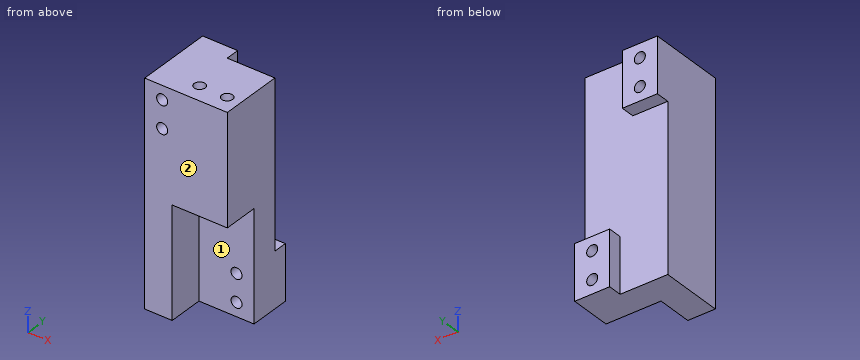
from build123d import *

# Parameters (mm, degrees)
SKETCH1_W           = 30
SKETCH1_H           = 80
BOSS_EXTRUDE1_DEPTH = 30
SKETCH2_W           = 12.7
SKETCH2_H           = 20
SKETCH2_R           = 2
BOSS_EXTRUDE2_DEPTH = 5
SKETCH3_R           = 2
CUT_EXTRUDE1_DEPTH  = 93.330926563
SKETCH4_W           = 20
SKETCH4_H           = 20
CUT_EXTRUDE2_DEPTH  = 40
SKETCH5_R           = 2
SKETCH5_W           = 30
SKETCH5_H           = 7.2
CUT_EXTRUDE3_DEPTH  = 93.330926563


with BuildPart() as part:
    # Sketch1 → Boss-Extrude1 (new body)
    with BuildSketch(Plane(origin=(0, 0, 0), x_dir=(1, 0, 0), z_dir=(0, 1, 0))):
        with Locations((-15, 40)):
            Rectangle(SKETCH1_W, SKETCH1_H)
    extrude(amount=BOSS_EXTRUDE1_DEPTH)

    # Sketch2 → Boss-Extrude2 (add)
    # profile 1 of 2: a face of its own
    with BuildSketch(Plane(origin=(0, 30, 0), x_dir=(1, 0, 0), z_dir=(0, 1, 0))):
        with Locations((-23.65, 10)):
            Rectangle(SKETCH2_W, SKETCH2_H)
        with Locations(Location((-23.65, 5, 0), (0, 0, 270))):
            Circle(SKETCH2_R, mode=Mode.SUBTRACT)
        with Locations(Location((-23.65, 15, 0), (0, 0, 270))):
            Circle(SKETCH2_R, mode=Mode.SUBTRACT)
    # profile 2 of 2: a face of its own
    with BuildSketch(Plane(origin=(0, 30, 0), x_dir=(1, 0, 0), z_dir=(0, 1, 0))):
        with Locations((-6.35, 70)):
            Rectangle(SKETCH2_W, SKETCH2_H)
        with Locations(Location((-6.35, 65, 0), (0, 0, 270))):
            Circle(SKETCH2_R, mode=Mode.SUBTRACT)
        with Locations(Location((-6.35, 75, 0), (0, 0, 270))):
            Circle(SKETCH2_R, mode=Mode.SUBTRACT)
    extrude(amount=BOSS_EXTRUDE2_DEPTH)

    # Sketch3 → Cut-Extrude1 (cut, through all)
    with BuildSketch(Plane(origin=(0, 35, 0), x_dir=(1, 0, 0), z_dir=(0, 1, 0))):
        with Locations(Location((-23.65, 15, 0), (0, 0, 270))):
            Circle(SKETCH3_R)
        with Locations(Location((-23.65, 5, 0), (0, 0, 270))):
            Circle(SKETCH3_R)
        with Locations(Location((-6.35, 75, 0), (0, 0, 270))):
            Circle(SKETCH3_R)
        with Locations(Location((-6.35, 65, 0), (0, 0, 270))):
            Circle(SKETCH3_R)
    extrude(amount=-CUT_EXTRUDE1_DEPTH, mode=Mode.SUBTRACT)

    # Sketch4 → Cut-Extrude2 (cut)
    with BuildSketch(Plane(origin=(0, 0, -80), x_dir=(-1, 0, 0), z_dir=(0, 0, -1))):
        with Locations((10, 10)):
            Rectangle(SKETCH4_W, SKETCH4_H)
    extrude(amount=-CUT_EXTRUDE2_DEPTH, mode=Mode.SUBTRACT)

    # Sketch5 → Cut-Extrude3 (cut, through all)
    with BuildSketch(Plane(origin=(0, 0, -80), x_dir=(-1, 0, 0), z_dir=(0, 0, -1))):
        with Locations((4.9, 13.6)):
            Circle(SKETCH5_R)
        with Locations((14.9, 13.6)):
            Circle(SKETCH5_R)
        with Locations((15, 3.6)):
            Rectangle(SKETCH5_W, SKETCH5_H)
    extrude(amount=-CUT_EXTRUDE3_DEPTH, mode=Mode.SUBTRACT)


solid = part.part
The model under review builds one solid part; all positions refer to its coordinate system, in mm. Face numbers are marked on the shaded views. A direction names the side the tool comes from. Give positions to 0.01 mm unless a question says otherwise; leave off trailing zeros. Write each loop counter-clockwise with the first axis right and the second up, starting at its lowest first coordinate (ties: lowest second). Pieces come first, ordered by that corner, then holes.
1. Add section C-C, the plane y = 13.6. Write out the cut boundary in (x, z), plus the area to 3 significant figures.
2. Add section D-D, the plane x = -14.9. Write out the cut boundary in (y, z).
3. For P1, Ø4, axis at x = -12.5, z = -48.5, coming from the +Y side; P2, Ø5, axis at y = 17, z = -31, coming from the +X side; P3, Ø5.5, axis at x = -8.5, y = 33, coming from the +Z side; P4, Ø2.5, axis at y = 33.5, z = -75, coming from the -X side, all flat-tipped, find the tip position at first contact; note any pin that passes through.
4. Wall thickness on L1, parallel to X at y = 19, z = -5; L2, parallel to Z at x = -7.5, y = 27.25; L3, parallel to X at y = 8.75, z = -62: over which ranges is each line inside the solid? List them lowest first.
5. Add section B-B, the plane z = -75. Write out the cut boundary in (x, y), plus the area to 4 significant figures.
6. Tool access review of the marked faces 1 and 2: name each direction out of +Z, -Z, +X, -X, +Y, -Y from which nothing blocks a thin tool from reaching the whole face with its end or side.
7. Add section A-A, the plane y = 25. Write out the cut boundary in (x, z), plus the area to 3 significant figures.
Worked answers:
1. outline: (-30, -80) - (-20, -80) - (-20, -40) - (-16.9, -40) - (-16.9, 0) - (-30, 0) - close; (-12.9, -40) - (-6.9, -40) - (-6.9, 0) - (-12.9, 0) - close; (-2.9, -40) - (0, -40) - (0, 0) - (-2.9, 0) - close; hole circle Ø4 at (-23.65, -15); hole circle Ø4 at (-23.65, -5)
1. area: 1,250 mm2
2. outline: (7.2, -40) - (11.6, -40) - (11.6, 0) - (7.2, 0) - close; (15.6, -40) - (20, -40) - (20, -80) - (30, -80) - (30, 0) - (15.6, 0) - close
3. P1: stops at y = 30
3. P2: stops at x = 0
3. P3: stops at z = -60
3. P4: stops at x = -12.7
4. L1: x = -30 to -25.65, -21.65 to 0
4. L2: z = -80 to -76.64, -73.36 to -66.64, -63.36 to 0
4. L3: x = -30 to -20
5. outline: (-30, 7.2) - (-20, 7.2) - (-20, 20) - (-8.35, 20) - (-8.35, 35) - (-12.7, 35) - (-12.7, 30) - (-30, 30) - close; (-4.35, 20) - (0, 20) - (0, 35) - (-4.35, 35) - close
5. area: 431.5 mm2
6. face 1: -Z, +X, -Y
6. face 2: +Z, -Z, +X, -X, -Y
7. outline: (-30, -80) - (0, -80) - (0, 0) - (-30, 0) - close; hole circle Ø4 at (-23.65, -15); hole circle Ø4 at (-23.65, -5); hole circle Ø4 at (-6.35, -75); hole circle Ø4 at (-6.35, -65)
7. area: 2,350 mm2
